from build123d import *

# Parameters (mm, degrees)
SKETCH1_W                = 1164
SKETCH1_H                = 396
BASE_PANEL_DEPTH         = 18
SKETCH2_R                = 4
EXTRUDE2_DEPTH           = 15
EXTRUDE3_START           = -15
SKETCH3_R                = 4
EXTRUDE3_DEPTH           = 15
SKETCH5_R                = 15
EXTRUDE17_DEPTH          = 13
TAGLIO_ESTRUSIONE1_START = -18
SKETCH4_2_R              = 4
TAGLIO_ESTRUSIONE1_DEPTH = 10


with BuildPart() as part:
    # Sketch1 → Base Panel (new body)
    with BuildSketch(Plane(origin=(0, -18, 0), x_dir=(-1, 0, 0), z_dir=(0, 1, 0))):
        with Locations((582, -198)):
            Rectangle(SKETCH1_W, SKETCH1_H)
    extrude(amount=BASE_PANEL_DEPTH)

    # Sketch2 → Extrude2 (cut)
    with BuildSketch(Plane(origin=(-1164, 0, 0), x_dir=(0, 0, -1), z_dir=(1, 0, 0))):
        with Locations((50, -11)):
            Circle(SKETCH2_R)
        with Locations((75, -11)):
            Circle(SKETCH2_R)
        with Locations((321, -11)):
            Circle(SKETCH2_R)
        with Locations((346, -11)):
            Circle(SKETCH2_R)
    extrude(amount=EXTRUDE2_DEPTH, mode=Mode.SUBTRACT)

    # Sketch3 → Extrude3 (cut)
    with BuildSketch(Plane(origin=(0, 0, 0), x_dir=(0, 0, -1), z_dir=(1, 0, 0)).offset(EXTRUDE3_START)):
        with Locations((346, -11)):
            Circle(SKETCH3_R)
        with Locations((321, -11)):
            Circle(SKETCH3_R)
        with Locations((75, -11)):
            Circle(SKETCH3_R)
        with Locations((50, -11)):
            Circle(SKETCH3_R)
    extrude(amount=EXTRUDE3_DEPTH, mode=Mode.SUBTRACT)

    # Sketch5 → Extrude17 (cut)
    with BuildSketch(Plane(origin=(0, -18, 0), x_dir=(-1, 0, 0), z_dir=(0, 1, 0))):
        with Locations(Location((25, -50, 0), (0, 0, 90))):
            Circle(SKETCH5_R)
        with Locations(Location((25, -346, 0), (0, 0, 90))):
            Circle(SKETCH5_R)
        with Locations(Location((1139, -50, 0), (0, 0, 90))):
            Circle(SKETCH5_R)
        with Locations(Location((1139, -346, 0), (0, 0, 90))):
            Circle(SKETCH5_R)
    extrude(amount=EXTRUDE17_DEPTH, mode=Mode.SUBTRACT)

    # Sketch4<2> → Taglio-Estrusione1 (cut)
    with BuildSketch(Plane(origin=(0, 0, 0), x_dir=(1, 0, 0), z_dir=(0, 1, 0)).offset(TAGLIO_ESTRUSIONE1_START)):
        with Locations(Location((-582, 15, 0), (0, 0, 270))):
            Circle(SKETCH4_2_R)
        with Locations(Location((-582, 60, 0), (0, 0, 270))):
            Circle(SKETCH4_2_R)
    extrude(amount=TAGLIO_ESTRUSIONE1_DEPTH, mode=Mode.SUBTRACT)


solid = part.part
Can you work these out from the model? Positions are in its coordinate system, mm. A direction names the side the tool comes from. Give positions to 0.01 mm unless a question says otherwise; leave off trailing zeros. Write each loop counter-clockwise with the first axis right and the second up, starting at its lowest first coordinate (ties: lowest second). Pieces come first, ordered by that corner, then holes. Notation, with made-up numbers: (70.25, 9) -> (85.25, 9) arc R15 cw to (85.25, 19) -> close; hole circle Ø7 at (59, 41.25). An arc over 180 degrees is marked (long way). Answer as a JSON object with one key per item and string values. Group by question number.
Item 1: I'm going to push flat-ended pins straight in: P1, Ø24, axis at x = -1137.5, z = -51, coming from the -Y side; P2, Ø4, axis at y = -12, z = -75, coming from the -X side; P3, Ø4, axis at y = -11.5, z = -321, coming from the +X side. Where does each tip first touch, or does it pass through?
Item 2: We'd pull the mould along X, two halves only. Please class faces 1 (the face through (-25, -5, -50)), 2 (the face through (-574, -18, -195)): +X half, -X half, draft (parallel to the pull), parting line (faces both ways), or undercut.
Item 3: For faces 3 (the face through (-574, 0, -195)), 4 (the face through (-25, -5, -346)), which set-ups out of +Z, -Z, +X, -X, +Y, -Y let a thin tool reach every point of the face, with its end or its side?
Item 4: Please list where these lines run through material, in increasing order: line 1 (Z direction, x = -582, y = -13); line 2 (X direction, y = -14.75, z = -15); line 3 (X direction, y = -14, z = -60). Write a range as [from, to].
Item 5: Suppose I cut it at A-A (x = -25). Please give me the cut outline in (y, z), plus the area to 3 significant figures.
Findings:
{
 "1": {"P1": "stops at y = -5", "P2": "stops at x = -1149", "P3": "stops at x = -15"},
 "2": {"face 1": "undercut", "face 2": "draft"},
 "3": {"face 3": "+Z, -Z, +X, -X, +Y", "face 4": "-Y"},
 "4": {"line 1": "z = [-396, -64], [-56, -19], [-11, 0]", "line 2": "x = [-1164, -586], [-578, 0]", "line 3": "x = [-1164, -1150.18], [-1127.82, -586], [-578, -36.18], [-13.82, 0]"},
 "5": {"outline": "(-18, -396) -> (0, -396) -> (0, 0) -> (-18, 0) -> (-18, -35) -> (-5, -35) -> (-5, -65) -> (-18, -65) -> (-18, -331) -> (-5, -331) -> (-5, -361) -> (-18, -361) -> close", "area": "6,350 mm²"}
}
